Design review of the part built by this model. Coordinates are the model's own, in mm. Coordinates: 2 decimals unless noted, no trailing zeros. Loops run counter-clockwise (first coordinate to the right, second up) from the corner with the lowest first, then second, coordinate; pieces in that order, holes last. Notation, with made-up numbers: (75, 63.25) -> (89, 63.25) arc R19 cw to (89, 73.25) -> close; hole circle Ø2 at (1.25, -29.75). An arc over 180 degrees is marked (long way). Use a Markdown table: item, result. Add a question column.
Q1. Take a section at A-A on z = 245. Count the separate pieces of the cut face and the enclosed holes in it, plus the area to 3 significant figures.
Q2. Clearance check with a flat-ended pin moving along its axis: pin 1 Ø2.5 at (x, y) = (246.65, 178.28) entering from -Z. State where the tip first meets the part, or that it passes through.
Q3. For probe 1 along X at (y, z) = (185.5, 243); probe 2 along Y at (x, z) = (205, 241.75); probe 3 along X at (y, z) = (177.5, 245), list the stretches that pass through material, from the lowest coordinate up.
Q4. Take a section at B-B on x = 230.5. Write out the cut boundary in (y, z), plus the area to 3 significant figures.
from build123d import *

# Parameters (mm, degrees)
BOSS_EXTRUDE1_DEPTH      = 60
BOSS_EXTRUDE1_DEPTH_BACK = 46
SKETCH2_R                = 1.7
CUT_EXTRUDE1_DEPTH       = 10


with BuildPart() as part:
    # Sketch1 → Boss-Extrude1 (new, two sides: drawn at the far end of the back side and taken through both)
    with BuildSketch(Plane(origin=(190.645148, 0, 0), x_dir=(0, 0, -1), z_dir=(1, 0, 0)).offset(-BOSS_EXTRUDE1_DEPTH_BACK)):
        with BuildLine():
            Line((-240.970904961, 189.163538159), (-246.970904961, 189.163538159))
            Line((-246.970904961, 189.163538159), (-246.970904961, 173.663538158))
            Line((-246.970904961, 173.663538158), (-240.970904961, 173.663538158))
            Line((-240.970904961, 173.663538158), (-240.970904961, 179.413538158))
            Line((-240.970904961, 179.413538158), (-241.970904961, 179.413538158))
            ThreePointArc((-241.970904961, 179.413538158), (-243.970904961, 181.413538158), (-241.970904961, 183.413538158))
            Line((-241.970904961, 183.413538158), (-240.970904961, 183.413538158))
            Line((-240.970904961, 183.413538158), (-240.970904961, 189.163538159))
        make_face()
    extrude(amount=BOSS_EXTRUDE1_DEPTH + BOSS_EXTRUDE1_DEPTH_BACK)

    # Sketch2 → Cut-Extrude1 (cut)
    with BuildSketch(Plane.XY.offset(246.970904961)):
        with BuildLine():
            ThreePointArc((176.345148, 178.278360264), (174.645148, 179.978360264), (172.945148, 178.278360264))
            ThreePointArc((172.945148, 178.278360264), (174.645148, 176.578360264), (176.345148, 178.278360264))
        make_face()
        with BuildLine():
            ThreePointArc((152.345148, 178.278360264), (149.443066472, 179.480441792), (150.645148, 176.578360264))
            Line((150.645148, 176.578360264), (150.645148, 178.278360264))
            Line((150.645148, 178.278360264), (152.345148, 178.278360264))
        make_face()
        with BuildLine():
            Line((150.645148, 178.278360264), (150.645148, 176.578360264))
            ThreePointArc((150.645148, 176.578360264), (151.847229528, 177.076278736), (152.345148, 178.278360264))
            Line((152.345148, 178.278360264), (150.645148, 178.278360264))
        make_face()
        with BuildLine():
            ThreePointArc((152.345148, 185.288538158), (150.645148, 186.988538158), (148.945148, 185.288538158))
            Line((148.945148, 185.288538158), (150.645148, 185.288538158))
            Line((150.645148, 185.288538158), (152.345148, 185.288538158))
        make_face()
        with BuildLine():
            Line((150.645148, 185.288538158), (148.945148, 185.288538158))
            ThreePointArc((148.945148, 185.288538158), (150.644787533, 183.588538197), (152.345147847, 185.287817224))
            Line((152.345147847, 185.287817224), (150.645148, 185.288538158))
        make_face()
        with BuildLine():
            Line((152.345148, 185.288538158), (150.645148, 185.288538158))
            Line((150.645148, 185.288538158), (152.345147847, 185.287817224))
            ThreePointArc((152.345147847, 185.287817224), (152.345147962, 185.288177691), (152.345148, 185.288538158))
        make_face()
        with BuildLine():
            ThreePointArc((176.345148, 185.278360264), (175.847229528, 186.480441792), (174.645148, 186.978360264))
            Line((174.645148, 186.978360264), (174.645148, 185.278360264))
            Line((174.645148, 185.278360264), (172.945148153, 185.279081198))
            ThreePointArc((172.945148153, 185.279081198), (174.644787533, 183.578360302), (176.345148, 185.278360264))
        make_face()
        with BuildLine():
            Line((174.645148, 185.278360264), (174.645148, 186.978360264))
            ThreePointArc((174.645148, 186.978360264), (173.446670303, 186.484034851), (172.945178468, 185.288538158))
            ThreePointArc((172.945178468, 185.288538158), (172.945156734, 185.283809699), (172.945148153, 185.279081198))
            Line((172.945148153, 185.279081198), (174.645148, 185.278360264))
        make_face()
        with Locations((198.645148, 178.278360264)):
            Circle(SKETCH2_R)
        with Locations((246.645148, 185.278360264)):
            Circle(SKETCH2_R)
        with Locations((246.645148, 178.278360264)):
            Circle(SKETCH2_R)
        with Locations((222.645148, 185.278360264)):
            Circle(SKETCH2_R)
        with Locations((222.645148, 178.278360264)):
            Circle(SKETCH2_R)
        with Locations((198.645148, 185.278360264)):
            Circle(SKETCH2_R)
    extrude(amount=-CUT_EXTRUDE1_DEPTH, mode=Mode.SUBTRACT)


solid = part.part
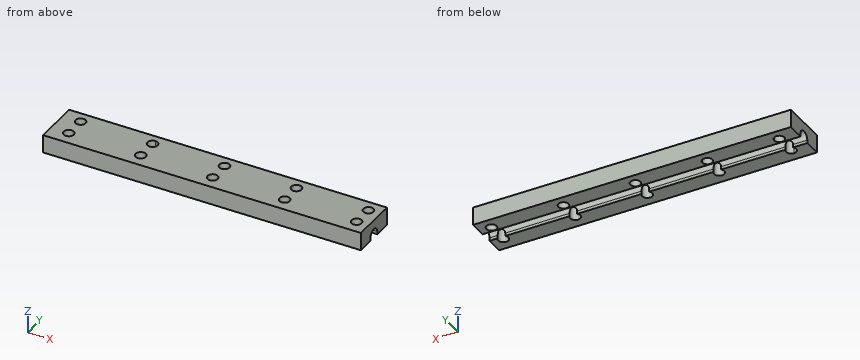
Answer list:
| question | item | result |
|---|---|---|
| 1 | separate pieces | 1 |
| 1 | enclosed holes | 10 |
| 1 | area | 1,550 mm² |
| 2 | pin 1 | through |
| 3 | probe 1 | 144.65 to 148.96, 152.33 to 172.96, 176.33 to 196.96, 200.33 to 220.96, 224.33 to 244.96, 248.33 to 250.65 |
| 3 | probe 2 | 173.66 to 179.41, 183.41 to 189.16 |
| 3 | probe 3 | 144.65 to 149.13, 152.16 to 173.13, 176.16 to 197.13, 200.16 to 221.13, 224.16 to 245.13, 248.16 to 250.65 |
| 4 | outline | (173.66, 240.97) -> (179.41, 240.97) -> (179.41, 241.97) arc R2 cw to (183.41, 241.97) -> (183.41, 240.97) -> (189.16, 240.97) -> (189.16, 246.97) -> (173.66, 246.97) -> close |
| 4 | area | 82.7 mm² |
